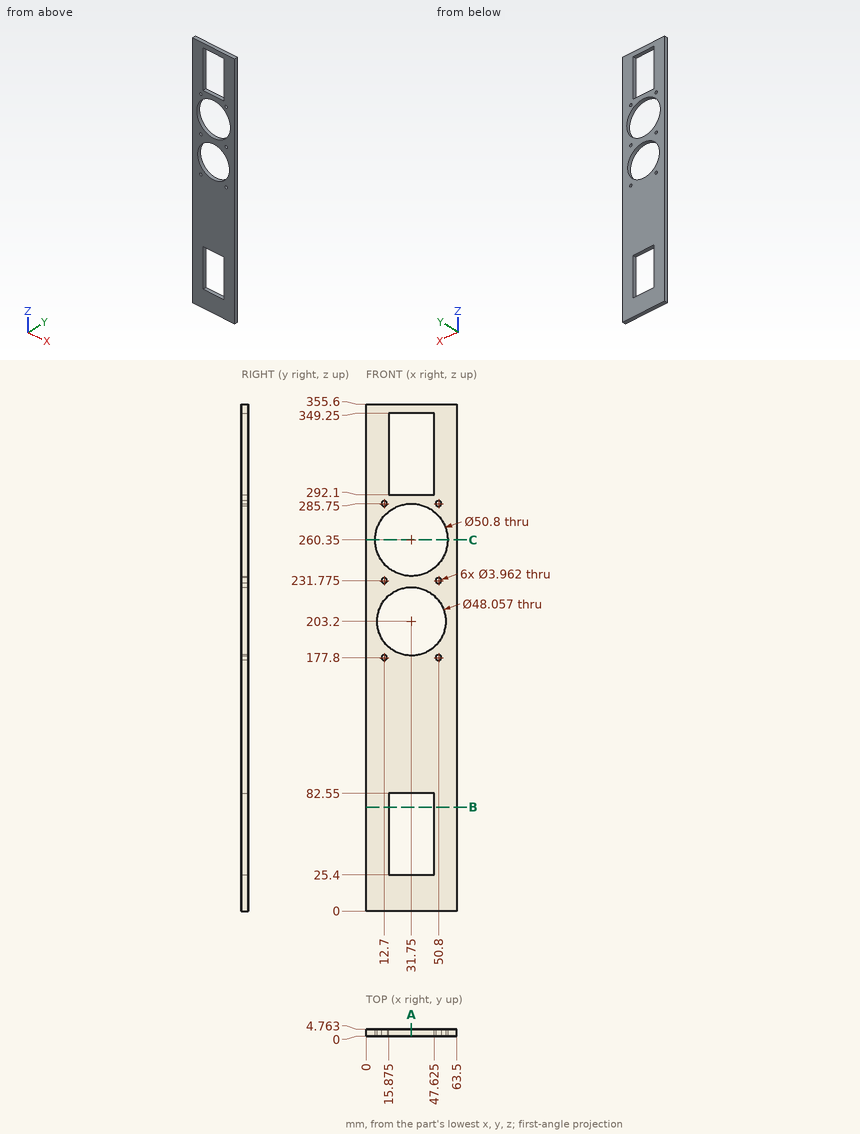
Can you work these out from the drawing? Everything is in mm from the part's minimum corner. Coordinates: 2 decimals unless noted, no trailing zeros. Loops run counter-clockwise (first coordinate to the right, second up) from the corner with the lowest first, then second, coordinate; pieces in that order, holes last.
1) Imagine slicing it at A-A (x = 31.75). List the corners of the cut face in (y, z) for me.
Reported:
outline: (0, 0) - (4.76, 0) - (4.76, 25.4) - (0, 25.4) - close; (0, 82.55) - (4.76, 82.55) - (4.76, 179.17) - (0, 179.17) - close; (0, 227.23) - (4.76, 227.23) - (4.76, 234.95) - (0, 234.95) - close; (0, 285.75) - (4.76, 285.75) - (4.76, 292.1) - (0, 292.1) - close; (0, 349.25) - (4.76, 349.25) - (4.76, 355.6) - (0, 355.6) - close
2) Will these pins go through, and if not, where does the flat tip stop? pin 1 Ø5 at (x, z) = (12.7, 285.75) entering from -Y; pin 2 Ø2.5 at (x, z) = (50.8, 231.775) entering from -Y.
Reported:
pin 1: stops at y = 0
pin 2: passes through
3) Imagine slicing it at B-B (z = 73). List the corners of the cut face in (x, y) for me (1 decimal).
Reported:
outline: (0, 0) - (15.9, 0) - (15.9, 4.8) - (0, 4.8) - close; (47.6, 0) - (63.5, 0) - (63.5, 4.8) - (47.6, 4.8) - close
4) Please list where these lines run through material, in increasing order: line 1 along Z through (x, y) = (31.75, 2.5); line 2 along X through (y, z) = (3.6, 177.8); line 3 along X through (y, z) = (0.3, 202.5).
Reported:
line 1: z = 0 to 25.4, 82.55 to 179.17, 227.23 to 234.95, 285.75 to 292.1, 349.25 to 355.6
line 2: x = 0 to 10.72, 14.68 to 48.82, 52.78 to 63.5
line 3: x = 0 to 7.73, 55.77 to 63.5
5) Imagine slicing it at C-C (z = 260.35). List the corners of the cut face in (x, y) for me.
Reported:
outline: (0, 0) - (6.35, 0) - (6.35, 4.76) - (0, 4.76) - close; (57.15, 0) - (63.5, 0) - (63.5, 4.76) - (57.15, 4.76) - close
